from build123d import *

# Parameters (mm, degrees)
SKETCH1_W           = 24
SKETCH1_H           = 13
BOSS_EXTRUDE1_DEPTH = 15
SKETCH2_W           = 20.15
SKETCH2_H           = 1.75
CUT_EXTRUDE1_DEPTH  = 15
FILLET1_R           = 2
CHAMFER2_SIZE       = 1
CHAMFER2_SIZE2      = 2.747477419
FILLET2_R           = 0.5
CUT_EXTRUDE4_DEPTH  = 11
SKETCH5_W           = 26.855674208
SKETCH5_H           = 19.307728506
CUT_EXTRUDE5_DEPTH  = 8
CUT_EXTRUDE6_DEPTH  = 11
SKETCH7_W           = 29.982721697
SKETCH7_H           = 21.559004648
CUT_EXTRUDE7_DEPTH  = 3
CHAMFER3_SIZE       = 2
FILLET3_R           = 0.4
FILLET4_R           = 0.2


with BuildPart() as part:
    # Sketch1 → Boss-Extrude1 (new body)
    with BuildSketch(Plane(origin=(0, 0, 0), x_dir=(1, 0, 0), z_dir=(0, 1, 0))):
        Rectangle(SKETCH1_W, SKETCH1_H)
    extrude(amount=BOSS_EXTRUDE1_DEPTH)

    # Sketch2 → Cut-Extrude1 (cut)
    with BuildSketch(Plane.XY.offset(6.5)):
        with Locations((0, 7.575)):
            Rectangle(SKETCH2_W, SKETCH2_H)
    extrude(amount=-CUT_EXTRUDE1_DEPTH, mode=Mode.SUBTRACT)

    # Fillet1
    fillet1_edges = [part.edges().sort_by_distance(p)[0] for p in [
        (-12, 15, 0),
        (12, 15, 0),
        (-12, 0, 0),
        (12, 0, 0),
    ]]
    fillet(fillet1_edges, radius=FILLET1_R)

    # Chamfer2
    chamfer2_edges = [part.edges().sort_by_distance(p)[0] for p in [
        (0, 15, 6.5),
        (12, 7.5, 6.5),
        (0, 0, 6.5),
        (-12, 7.5, 6.5),
        (-11.414213562, 14.414213562, 6.5),
        (-11.414213562, 0.585786438, 6.5),
        (11.414213562, 0.585786438, 6.5),
        (11.414213562, 14.414213562, 6.5),
    ]]
    chamfer2_side = [part.faces().sort_by_distance(p)[0] for p in [
        (11.716980566, 7.5, 6.5),
    ]]
    chamfer(chamfer2_edges, length=CHAMFER2_SIZE, length2=CHAMFER2_SIZE2, reference=chamfer2_side[0])

    # Fillet2
    fillet2_edges = [part.edges().sort_by_distance(p)[0] for p in [
        (10.075, 7.575, 6.5),
        (0, 8.45, 6.5),
        (-10.075, 7.575, 6.5),
        (0, 6.7, 6.5),
    ]]
    fillet(fillet2_edges, radius=FILLET2_R)

    # Sketch4 → Cut-Extrude4 (cut)
    with BuildSketch(Plane(origin=(0, 0, -6.5), x_dir=(-1, 0, 0), z_dir=(0, 0, -1))):
        Polygon((-10.075, 8.45), (-8.575, 8.45), (-8.575, 11.891155889), (8.575, 11.891155889), (8.575, 8.45), (10.075, 8.45), (10.075, 6.7), (-10.075, 6.7), align=None)
    extrude(amount=-CUT_EXTRUDE4_DEPTH, mode=Mode.SUBTRACT)

    # Sketch5 → Cut-Extrude5 (cut)
    with BuildSketch(Plane(origin=(0, 0, -6.5), x_dir=(-1, 0, 0), z_dir=(0, 0, -1))):
        with Locations((-0.083402715, 7.762018115)):
            Rectangle(SKETCH5_W, SKETCH5_H)
        with BuildLine():
            Line((10, 14), (-10, 14))
            ThreePointArc((-10, 14), (-10.707106781, 13.707106781), (-11, 13))
            Line((-11, 13), (-11, 2))
            ThreePointArc((-11, 2), (-10.707106781, 1.292893219), (-10, 1))
            Line((-10, 1), (10, 1))
            ThreePointArc((10, 1), (10.707106781, 1.292893219), (11, 2))
            Line((11, 2), (11, 13))
            ThreePointArc((11, 13), (10.707106781, 13.707106781), (10, 14))
        make_face(mode=Mode.SUBTRACT)
    extrude(amount=-CUT_EXTRUDE5_DEPTH, mode=Mode.SUBTRACT)

    # Sketch6 → Cut-Extrude6 (cut)
    with BuildSketch(Plane(origin=(0, 0, -6.5), x_dir=(-1, 0, 0), z_dir=(0, 0, -1))):
        with BuildLine():
            Line((-9, 5.7), (9, 5.7))
            ThreePointArc((9, 5.7), (9.707106781, 5.407106781), (10, 4.7))
            Line((10, 4.7), (10, 3))
            ThreePointArc((10, 3), (9.707106781, 2.292893219), (9, 2))
            Line((9, 2), (-9, 2))
            ThreePointArc((-9, 2), (-9.707106781, 2.292893219), (-10, 3))
            Line((-10, 3), (-10, 4.7))
            ThreePointArc((-10, 4.7), (-9.707106781, 5.407106781), (-9, 5.7))
        make_face()
    extrude(amount=-CUT_EXTRUDE6_DEPTH, mode=Mode.SUBTRACT)

    # Sketch7 → Cut-Extrude7 (cut)
    with BuildSketch(Plane(origin=(0, 0, -6.5), x_dir=(-1, 0, 0), z_dir=(0, 0, -1))):
        with Locations((0.615824589, 7.279559508)):
            Rectangle(SKETCH7_W, SKETCH7_H)
    extrude(amount=-CUT_EXTRUDE7_DEPTH, mode=Mode.SUBTRACT)

    # Chamfer3
    chamfer3_edges = [part.edges().sort_by_distance(p)[0] for p in [
        (9.325, 8.45, -3.5),
        (-9.325, 8.45, -3.5),
    ]]
    chamfer(chamfer3_edges, length=CHAMFER3_SIZE)

    # Fillet3
    fillet3_edges = [part.edges().sort_by_distance(p)[0] for p in [
        (-10, 3.85, -3.5),
        (0, 14, -3.5),
        (-10.707106781, 13.707106781, -3.5),
        (-11, 7.5, -3.5),
        (-10.707106781, 1.292893219, -3.5),
        (0, 1, -3.5),
        (10.707106781, 1.292893219, -3.5),
        (11, 7.5, -3.5),
        (10.707106781, 13.707106781, -3.5),
        (0, 6.7, -3.5),
        (0, 11.891155889, -3.5),
        (-8.575, 11.170577944, -3.5),
        (-9.707106781, 2.292893219, -3.5),
        (0, 2, -3.5),
        (9.707106781, 2.292893219, -3.5),
        (10, 3.85, -3.5),
        (9.707106781, 5.407106781, -3.5),
        (0, 5.7, -3.5),
        (-9.707106781, 5.407106781, -3.5),
        (8.575, 11.170577944, -3.5),
        (-9.325, 10.45, -3.5),
        (9.325, 10.45, -3.5),
    ]]
    fillet(fillet3_edges, radius=FILLET3_R)

    # Fillet4
    fillet4_edges = [part.edges().sort_by_distance(p)[0] for p in [
        (-11.414213562, 14.414213562, 1.5),
        (0, 0, 1.5),
        (-12, 7.5, 1.5),
        (12, 7.5, 1.5),
        (11.414213562, 0.585786438, 1.5),
        (11.414213562, 14.414213562, 1.5),
        (0, 15, 1.5),
        (-11.414213562, 0.585786438, 1.5),
    ]]
    fillet(fillet4_edges, radius=FILLET4_R)


solid = part.part
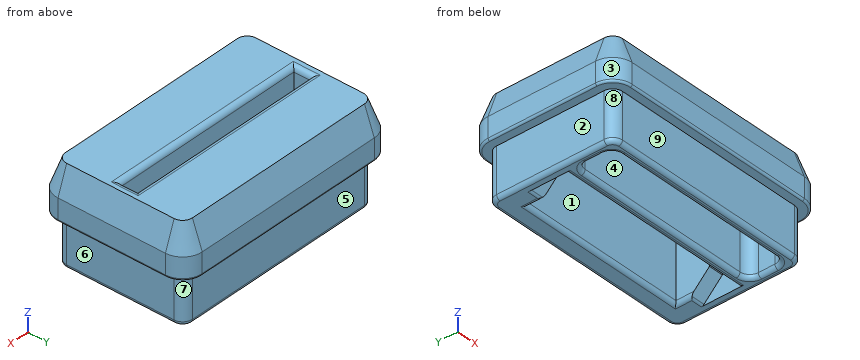
Check sheet for the modelled part. Datum: model origin and axes. Units: mm. Face numbers are marked on the shaded views. A direction names the side the tool comes from. Round coordinates to 2 decimals unless told otherwise and drop trailing zeros. Order: outer loops, then holes, each group sorted by start corner. A loop starts at its lowest first (then second) coordinate and runs counter-clockwise, first axis right, second up. Notation, with made-up numbers: M 17.25,19.25 L 22.25,19.25 A29 ccw 22.25,52.25 Z; hole C 55,55 d9. An arc over 180 degrees is marked long. One line per item, written item: value. Start each with the question number.
1. Section check C-C on y = 7.25. Enter the section's corners in (x, z) (3 decimals), and give its area (3 significant figures).
2. Gauge pin test, flat ends, axial feed: P1, Ø1.4, axis at x = 4.5, z = -0.5, coming from the +Y side; P2, Ø3.5, axis at y = 9, z = -1, coming from the +X side; P3, Ø0.8, axis at y = 4, z = 0.5, coming from the -X side. Record the tip position at first contact, or that the pin passes through.
3. Release check for a two-part mould opening along Y. For the marked faces 1, 2, 3 and 4 record: released by +Y, released by -Y, zero draft, split by the parting line, or undercut.
4. Section check D-D on z = 5. Enter the section's corners in (x, y) (3 decimals), and give its area (3 significant figures).
5. Access from +Z, -Z, +X, -X, +Y, -Y to the whole of each face (thin tool, end or side, straight path). Record for the marked faces 5, 6, 7, 8 and 9.
6. Section check A-A on z = 3.25. Enter the section's corners in (x, y) (3 decimals), and give its area (3 significant figures).
7. Scan lines: line 1 along Y through (x, z) = (0.5, -2); line 2 along Y through (x, z) = (-3.5, 3.5); line 3 along X through (y, z) = (11.75, -2) (3 decimals). Record each from-to range of solid material in increasing order.
Results found:
1. outline: M -12,1.7 A0.2 ccw -11.8,1.5 L -11,1.5 L -11,-3.1 A0.4 ccw -10.6,-3.5 L -10.075,-3.5 L -10.075,6 A0.5 ccw -10.575,6.5 L -11,6.5 L -12,3.753 Z; M 10.075,-3.5 L 10.6,-3.5 A0.4 ccw 11,-3.1 L 11,1.5 L 11.8,1.5 A0.2 ccw 12,1.7 L 12,3.753 L 11,6.5 L 10.575,6.5 A0.5 ccw 10.075,6 Z
1. area: 25.6 mm^2
2. P1: y = 14
2. P2: x = 11
2. P3: x = -11
3. face 1: undercut
3. face 2: zero draft
3. face 3: released by -Y
3. face 4: undercut
4. outline: M -11.546,2 A1.546 ccw -10,0.454 L 10,0.454 A1.546 ccw 11.546,2 L 11.546,13 A1.546 ccw 10,14.546 L -10,14.546 A1.546 ccw -11.546,13 Z; hole M -10.075,6.7 L 10.075,6.7 L 10.075,8.45 L -10.075,8.45 Z
4. area: 288 mm^2
5. face 5: -Z, +X, -X, +Y
5. face 6: -Z, +X, +Y, -Y
5. face 7: -Z, +X, +Y
5. face 8: -Z, -X, -Y
5. face 9: -Z, +X, -X, -Y
6. outline: M -12,2 A2 ccw -10,0 L 10,0 A2 ccw 12,2 L 12,13 A2 ccw 10,15 L -10,15 A2 ccw -12,13 Z; hole M -10.075,6.7 L 10.075,6.7 L 10.075,8.45 L 8.575,8.45 L 8.575,11.891 L -8.575,11.891 L -8.575,8.45 L -10.075,8.45 Z; hole M -10,3 A1 ccw -9,2 L 9,2 A1 ccw 10,3 L 10,4.7 A1 ccw 9,5.7 L -9,5.7 A1 ccw -10,4.7 Z
6. area: 189 mm^2
7. line 1: 1 to 2, 5.7 to 6.7, 11.89 to 14
7. line 2: 0 to 2, 5.7 to 6.7, 11.89 to 15
7. line 3: -11 to -8.575, 8.575 to 11
